Work out the finished part from the listing and answer in its coordinate system (mm). Face numbers are marked on the shaded views. A direction names the side the tool comes from. Round coordinates to 2 decimals unless told otherwise and drop trailing zeros. Loops run counter-clockwise (first coordinate to the right, second up) from the corner with the lowest first, then second, coordinate; pieces in that order, holes last. Notation, with made-up numbers: (35, 12.25) - (72, 12.25) arc R19 cw to (72, 21.25) - close; hole circle Ø4 at (2.5, -32). An arc over 180 degrees is marked (long way). Return JSON: item names as keys, results as strings.
from build123d import *

# Parameters (mm, degrees)
BOSS_EXTRUDE1_DEPTH = 20
SKETCH2_W           = 30
SKETCH2_H           = 25
CUT_EXTRUDE1_DEPTH  = 12
SKETCH5_R           = 2.75
CUT_EXTRUDE4_DEPTH  = 31
SKETCH6_R           = 6.7
CUT_EXTRUDE5_DEPTH  = 5
SKETCH7_R           = 2.5
CUT_EXTRUDE6_DEPTH  = 16


with BuildPart() as part:
    # Sketch1 → Boss-Extrude1 (new body)
    with BuildSketch(Plane(origin=(0, 0, 0), x_dir=(1, 0, 0), z_dir=(0, 1, 0))):
        Polygon((0, 0), (60, 0), (60, 35), (20, 35), (20, 15), (0, 15), align=None)
    extrude(amount=BOSS_EXTRUDE1_DEPTH)

    # Sketch2 → Cut-Extrude1 (cut)
    with BuildSketch(Plane(origin=(0, 20, 0), x_dir=(1, 0, 0), z_dir=(0, 1, 0))):
        with Locations((45, 22.5)):
            Rectangle(SKETCH2_W, SKETCH2_H)
    extrude(amount=-CUT_EXTRUDE1_DEPTH, mode=Mode.SUBTRACT)

    # Sketch5 → Cut-Extrude4 (cut, through all)
    with BuildSketch(Plane(origin=(30, 0, 0), x_dir=(0, 0, -1), z_dir=(1, 0, 0))):
        with Locations((25, 14)):
            Circle(SKETCH5_R)
    extrude(amount=-CUT_EXTRUDE4_DEPTH, mode=Mode.SUBTRACT)

    # Sketch6 → Cut-Extrude5 (cut)
    with BuildSketch(Plane.XZ):
        with Locations((46.1, -12.525762493)):
            Circle(SKETCH6_R)
    extrude(amount=-CUT_EXTRUDE5_DEPTH, mode=Mode.SUBTRACT)

    # Sketch7 → Cut-Extrude6 (cut, through all)
    with BuildSketch(Plane.XZ.offset(-5)):
        with Locations((46.1, -12.525762493)):
            Circle(SKETCH7_R)
    extrude(amount=-CUT_EXTRUDE6_DEPTH, mode=Mode.SUBTRACT)


solid = part.part
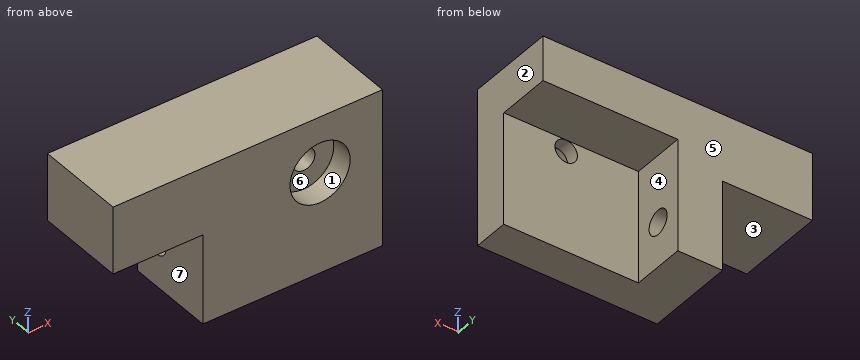
1) Determine the mould class of the marked faces 1, 2 and 3 for opening direction Z: pulls with the +Z half, pulls with the -Z half, needs draft (parallel to the pull), parting line crosses it, or undercut.
Verdict:
{"face 1": "undercut", "face 2": "needs draft", "face 3": "pulls with the -Z half"}
2) Section B-B (z = -25) is taken. Give the vertices of the cut face in (x, y), and give its area (3 significant figures).
Verdict:
{"outline": "(20, 0) - (60, 0) - (60, 8) - (30, 8) - (30, 11.25) - (20, 11.25) - close; (20, 16.75) - (30, 16.75) - (30, 20) - (20, 20) - close", "area": "385 mm2"}
3) A tool of negligible diameter and unlimited length cuts with its end or side. For the marked faces 4, 5, 6 and 7, from which of +Z, -Z, +X, -X, +Y, -Y can it reach the whole face along a straight path? Write none if from no direction.
Verdict:
{"face 4": "-Z, +X, +Y", "face 5": "+Z, -Z, +X, -X, +Y", "face 6": "-Y", "face 7": "-Z, -X, +Y, -Y"}
4) Flat-ended cylindrical pins translate along their axes: pin 1 (8 mm diameter, centred on x = 34.5, z = -26.5, fed in from +Y); pin 2 (4 mm diameter, centred on x = 45, z = -14, fed in from -Y); pin 3 (3 mm diameter, centred on x = 17, y = 11, fed in from -Z). Find the tip coordinate at first contact, or state that the pin passes through.
Verdict:
{"pin 1": "stops at y = 8", "pin 2": "stops at y = 5", "pin 3": "stops at z = -15"}
5) Find the intervals of material crossed by L1, parallel to Z at x = 46.1, y = 7.15; L2, parallel to Y at x = 22.5, z = -25; L3, parallel to Y at x = 34, z = -27.5, in increasing order.
Verdict:
{"L1": "z = -35 to -15.03, -10.03 to 0", "L2": "y = 0 to 11.25, 16.75 to 20", "L3": "y = 0 to 8"}
6) Section C-C (x = 46.5) is taken. Give the vertices of the cut face in (y, z), and give its area (3 significant figures).
Verdict:
{"outline": "(0, -35) - (8, -35) - (8, -14.99) - (5, -14.99) - (5, -19.21) - (0, -19.21) - close; (0, -5.84) - (5, -5.84) - (5, -10.06) - (8, -10.06) - (8, -10) - (20, -10) - (20, 0) - (0, 0) - close", "area": "318 mm2"}
7) Section A-A (y = 14) is taken. Give the vertices of the cut face in (x, z), and give its area (3 significant figures).
Verdict:
{"outline": "(0, -15) - (20, -15) - (20, -22.25) - (30, -22.25) - (30, -10) - (60, -10) - (60, 0) - (0, 0) - close; (20, -35) - (30, -35) - (30, -27.75) - (20, -27.75) - close", "area": "895 mm2"}
8) Section D-D (y = 6.5) is taken. Give the vertices of the cut face in (x, z).
Verdict:
{"outline": "(0, -15) - (20, -15) - (20, -35) - (60, -35) - (60, 0) - (0, 0) - close; hole circle Ø5 at (46.1, -12.53)"}
